Here's how the part is built. I have some questions about the finished solid (model axes, mm). A direction names the side the tool comes from. Give positions to 0.01 mm unless a question says otherwise; leave off trailing zeros. Loops run counter-clockwise (first coordinate to the right, second up) from the corner with the lowest first, then second, coordinate; pieces in that order, holes last. Notation, with made-up numbers: M 35,40.5 L 48,40.5 A15 ccw 48,66.5 Z; hole C 65.25,12.5 d3. An arc over 180 degrees is marked long. Write item = value, one per line. Start each with the question number.
```python
from build123d import *

# Parameters (mm, degrees)
F0_R     = 25.4
F1_DEPTH = 19.05
F2_R     = 5.08
F4_START = 12.7
F3_R     = 12.7
F3_R_2   = 6.35
F4_DEPTH = 12.7
F5_R     = 2.54
F6_R     = 3.96875
F7_DEPTH = 19.051


with BuildPart() as f1:
    # F0 (on Front) → F1 (new body)
    with BuildSketch(Plane.XZ):
        Circle(F0_R)
    extrude(amount=F1_DEPTH)

    # F2
    f2_edges = [f1.edges().sort_by_distance(p)[0] for p in [
        (-25.4, -19.05, 0),
        (-25.4, 0, 0),
    ]]
    fillet(f2_edges, radius=F2_R)

    # F3 (on Front) → F4 (cut)
    with BuildSketch(Plane.XZ.offset(F4_START)):
        Circle(F3_R)
        Circle(F3_R_2, mode=Mode.SUBTRACT)
    extrude(amount=F4_DEPTH, mode=Mode.SUBTRACT)

    # F5
    f5_edges = [f1.edges().sort_by_distance(p)[0] for p in [
        (-6.35, -19.05, 0),
        (-12.7, -19.05, 0),
    ]]
    fillet(f5_edges, radius=F5_R)

    # F6 (on Front) → F7 (cut, through all)
    with BuildSketch(Plane.XZ):
        Circle(F6_R)
    extrude(amount=F7_DEPTH, mode=Mode.SUBTRACT)


solid = f1.part
```
Q1. If we section it at A-A, the plane x = 0: List the corners of the cut face in (y, z) for me, then the cut area to 3 significant figures.
Q2. If we section it at D-D, the plane y = -6: List the corners of the cut face in (x, z) for me.
Q3. On a 3-axis mill with a long thin cutter (end or side, diameter ignored), from which of +Z, -Z, +X, -X, +Y, -Y can I reach the whole of each face in a straight line? I mean faces 4 (the cylindrical face through (-2.75, -14.58, -12.4)), 5 (the flat face through (2.92, -19.05, 15.15)). Say none if no direction works.
Q4. We'd pull the mould along X, two halves only. Please class faces 1 (the cylindrical face through (-5.506, -9.463, -24.796)), 2 (the cylindrical face through (-1.38, -14.58, -6.2)), 3 (the flat face through (4.2, 0, 0.3)): pulls with the +X half, pulls with the -X half, needs draft (parallel to the pull), parting line crosses it, or undercut.
Q5. If we section it at C-C, the plane y = -15.25: List the corners of the cut face in (x, z) for me, then the cut area to 3 significant figures.
Q6. Will these pins go through, and if not, where does the flat tip stop? pin 1 (4 mm diameter, centred on x = -1, y = -4, fed in from +Z); pin 2 (1 mm diameter, centred on x = -13.5, z = -5, fed in from -Y); pin 3 (6 mm diameter, centred on y = -4.5, z = 15, fed in from -X); pin 4 (5 mm diameter, centred on x = 0, z = 0, fed in from -Y).
Q7. If we section it at B-B, the plane z = 0: List the corners of the cut face in (x, y) for me.
Q8. If I drill on line 1 along Z through (x, y) = (0, -14); line 2 along Z through (x, y) = (0, -15.55); line 3 along Z through (x, y) = (0, -6.5), over which ranges is the centre line in solid material (lowest first)?
Resolved:
q1.outline = M -19.05,-20.32 A5.08 ccw -13.97,-25.4 L -5.08,-25.4 A5.08 ccw 0,-20.32 L 0,-3.97 L -19.05,-3.97 A2.54 ccw -16.51,-6.35 L -12.7,-6.35 L -12.7,-12.7 L -16.51,-12.7 A2.54 ccw -19.05,-15.24 Z; M -19.05,3.97 L 0,3.97 L 0,20.32 A5.08 ccw -5.08,25.4 L -13.97,25.4 A5.08 ccw -19.05,20.32 L -19.05,15.24 A2.54 ccw -16.51,12.7 L -12.7,12.7 L -12.7,6.35 L -16.51,6.35 A2.54 ccw Z
q1.area = 708 mm²
q2.outline = C 0,0 d50.8; hole C 0,0 d7.94
q3.face_4 = -Y
q3.face_5 = +Z, -Z, +X, -X, -Y
q4.face_1 = parting line crosses it
q4.face_2 = undercut
q4.face_3 = needs draft
q5.outline = C 0,0 d50.47; C 0,0 d12.7; hole C 0,0 d25.4; hole C 0,0 d7.94
q5.area = 1,570 mm²
q6.pin_1 = 25.4
q6.pin_2 = -19.03
q6.pin_3 = -22.37
q6.pin_4 = through
q7.outline = M -25.4,-13.97 A5.08 ccw -20.32,-19.05 L -15.24,-19.05 A2.54 ccw -12.7,-16.51 L -12.7,-12.7 L -6.35,-12.7 L -6.35,-16.51 A2.54 ccw -3.97,-19.05 L -3.97,0 L -20.32,0 A5.08 ccw -25.4,-5.08 Z; M 3.97,-19.05 A2.54 ccw 6.35,-16.51 L 6.35,-12.7 L 12.7,-12.7 L 12.7,-16.51 A2.54 ccw 15.24,-19.05 L 20.32,-19.05 A5.08 ccw 25.4,-13.97 L 25.4,-5.08 A5.08 ccw 20.32,0 L 3.97,0 Z
q8.line_1 = -25.4 to -12.7, -6.35 to -3.97, 3.97 to 6.35, 12.7 to 25.4
q8.line_2 = -25.15 to -12.7, -6.35 to -3.97, 3.97 to 6.35, 12.7 to 25.15
q8.line_3 = -25.4 to -3.97, 3.97 to 25.4
